Build history of the part. All positions in model axes, mm. A direction names the side the tool comes from. Round coordinates to 2 decimals unless told otherwise and drop trailing zeros. Write each loop counter-clockwise with the first axis right and the second up, starting at its lowest first coordinate (ties: lowest second). Pieces come first, ordered by that corner, then holes. Notation, with made-up numbers: (72, 8.25) -> (114, 8.25) arc R17 ccw to (114, 40.25) -> close; hole circle Ø10 at (-27.75, 54). An arc over 180 degrees is marked (long way). Return JSON: item names as keys, results as strings.
from build123d import *

# Parameters (mm, degrees)
F0_W     = 16
F0_H     = 20
F0_R     = 2.6
F0_R_2   = 1.25
F1_DEPTH = 11.6
F3_DEPTH = 16.001
F4_R     = 1.25
F5_DEPTH = 5
F6_SIZE  = 0.5


with BuildPart() as f1:
    # F0 (on Top) → F1 (new body)
    with BuildSketch(Plane.XY):
        with Locations((8, 10)):
            Rectangle(F0_W, F0_H)
        with Locations((8, 4.5)):
            Circle(F0_R, mode=Mode.SUBTRACT)
        with Locations((8, 17.5)):
            Circle(F0_R_2, mode=Mode.SUBTRACT)
    extrude(amount=F1_DEPTH)

    # F2 (on face) → F3 (cut, through all)
    with BuildSketch(Plane.YZ.offset(16)):
        with BuildLine():
            Line((21.9580398915, 7.85), (14.9580398915, 7.85))
            ThreePointArc((14.9580398915, 7.85), (9, 7.35), (14.9580398915, 6.85))
            Line((14.9580398915, 6.85), (21.9580398915, 6.85))
            Line((21.9580398915, 6.85), (21.9580398915, 7.85))
        make_face()
    extrude(amount=-F3_DEPTH, mode=Mode.SUBTRACT)

    # F4 (on face) → F5 (cut)
    with BuildSketch(Plane.YZ.offset(16)):
        with Locations((2, 9.6)):
            Circle(F4_R)
        with Locations((3.5, 5.6)):
            Circle(F4_R)
    extrude(amount=-F5_DEPTH, mode=Mode.SUBTRACT)

    # F6
    f6_edges = [f1.edges().sort_by_distance(p)[0] for p in [
        (0, 0, 5.8),
        (16, 0, 5.8),
        (8, 0, 0),
        (8, 0, 11.6),
        (16, 10, 11.6),
        (16, 10, 0),
        (16, 20, 3.425),
        (16, 20, 9.725),
        (0, 20, 9.725),
        (8, 20, 11.6),
        (8, 20, 0),
        (0, 20, 3.425),
        (0, 10, 11.6),
        (0, 10, 0),
    ]]
    chamfer(f6_edges, length=F6_SIZE)


solid = f1.part
Q1. Saw through at A-A on x = 7. List the corners of the cut face in (y, z), then the cut area to 3 significant figures.
Verdict:
{"outline": "(0, 0.5) -> (0.5, 0) -> (2.1, 0) -> (2.1, 11.6) -> (0.5, 11.6) -> (0, 11.1) -> close; (6.9, 0) -> (16.75, 0) -> (16.75, 6.85) -> (14.96, 6.85) arc R3 cw (long way) to (14.96, 7.85) -> (16.75, 7.85) -> (16.75, 11.6) -> (6.9, 11.6) -> close; (18.25, 0) -> (19.5, 0) -> (20, 0.5) -> (20, 6.85) -> (18.25, 6.85) -> close; (18.25, 7.85) -> (20, 7.85) -> (20, 11.1) -> (19.5, 11.6) -> (18.25, 11.6) -> close", "area": "127 mm²"}
Q2. 3-axis set-ups, long thin cutter, end or side, ignore diameter. For faces 1 (the flat face through (11, 2, 10)), 2 (the flat face through (0, 9.9, 4.5)), 3 (the flat face through (8, 19, 7.85)): which of +Z, -Z, +X, -X, +Y, -Y reach the whole face in a straight line?
Verdict:
{"face 1": "+X", "face 2": "+Z, -Z, -X, +Y, -Y", "face 3": "+X, -X, +Y"}
Q3. Pin check, flat tips, straight feed: pin 1 Ø0.8 at (y, z) = (4, 5.5) entering from +X; pin 2 Ø1.5 at (x, y) = (8, 17.5) entering from -Z. Stop position of each tip, or through.
Verdict:
{"pin 1": "stops at x = 11", "pin 2": "passes through"}
Q4. Saw through at C-C on z = 9.6. List the corners of the cut face in (x, y), then the cut area to 3 significant figures.
Verdict:
{"outline": "(0, 0.5) -> (0.5, 0) -> (15.5, 0) -> (16, 0.5) -> (16, 0.75) -> (11, 0.75) -> (11, 3.25) -> (16, 3.25) -> (16, 10.02) -> (0, 10.02) -> close; (0, 13.98) -> (16, 13.98) -> (16, 19.5) -> (15.5, 20) -> (0.5, 20) -> (0, 19.5) -> close; hole circle Ø5.2 at (8, 4.5); hole circle Ø2.5 at (8, 17.5)", "area": "217 mm²"}
Q5. Saw through at B-B on y = 3.5. List the corners of the cut face in (x, z).
Verdict:
{"outline": "(0, 0.5) -> (0.5, 0) -> (5.6, 0) -> (5.6, 11.6) -> (0.5, 11.6) -> (0, 11.1) -> close; (10.4, 0) -> (15.5, 0) -> (16, 0.5) -> (16, 4.35) -> (11, 4.35) -> (11, 6.85) -> (16, 6.85) -> (16, 11.1) -> (15.5, 11.6) -> (10.4, 11.6) -> close"}
Q6. Wall check: L1, parallel to Y at x = 8, z = 4.25; L2, parallel to Y at x = 9, z = 8; L3, parallel to Z at x = 6.25, y = 12. Give the ranges that are in metal, low to high.
Verdict:
{"L1": "y = 0 to 1.9, 7.1 to 16.25, 18.75 to 20", "L2": "y = 0 to 2.1, 6.9 to 9.07, 14.93 to 16.75, 18.25 to 20", "L3": "z = 0 to 4.35, 10.35 to 11.6"}
Q7. Two-plate mould, pull along X, no slides. Class faces 4 (the flat face through (11, 3, 6)), 5 (the flat face through (8, 16, 6.85)), 6 (the cylindrical face through (6.75, 17.55, 9.7)): +X half, -X half, draft (parallel to the pull), parting line (faces both ways), or undercut.
Verdict:
{"face 4": "+X half", "face 5": "draft", "face 6": "undercut"}
Q8. Saw through at D-D on y = 17.5. List the corners of the cut face in (x, z).
Verdict:
{"outline": "(0, 0.5) -> (0.5, 0) -> (6.75, 0) -> (6.75, 6.85) -> (0, 6.85) -> close; (0, 7.85) -> (6.75, 7.85) -> (6.75, 11.6) -> (0.5, 11.6) -> (0, 11.1) -> close; (9.25, 0) -> (15.5, 0) -> (16, 0.5) -> (16, 6.85) -> (9.25, 6.85) -> close; (9.25, 7.85) -> (16, 7.85) -> (16, 11.1) -> (15.5, 11.6) -> (9.25, 11.6) -> close"}
